The model under review builds one solid part; all positions refer to its coordinate system, in mm. Face numbers are marked on the shaded views. A direction names the side the tool comes from. Round coordinates to 2 decimals unless told otherwise and drop trailing zeros. Write each loop counter-clockwise with the first axis right and the second up, starting at its lowest first coordinate (ties: lowest second). Pieces come first, ordered by that corner, then holes. Notation, with made-up numbers: (29.5, -28) -> (68.5, -28) arc R15 ccw to (68.5, 0) -> close; hole circle Ø6 at (-6, 73.5). An arc over 180 degrees is marked (long way). Return JSON: item names as keys, results as strings. Group by question number.
1. Mouldability with a two-part tool opening along Z and no side actions: class the marked faces 1, 2 and 3 as pulls with the +Z half, pulls with the -Z half, needs draft (parallel to the pull), parting line crosses it, or undercut.
2. Take a section at C-C, the plane y = 2.45. Write out the cut boundary in (x, z).
3. Tool access review of the marked faces 4 and 5: name each direction out of +Z, -Z, +X, -X, +Y, -Y from which nothing blocks a thin tool from reaching the whole face with its end or side.
4. Take a section at D-D, the plane x = -7.25. Write out the cut boundary in (y, z), then the cut area to 3 significant figures.
5. For line 1 along X through (y, z) = (1.25, 0); line 2 along X through (y, z) = (0.7, 0.5); line 3 along Z through (x, y) = (-2.25, 2.5), list the stretches that pass through material, from the lowest coordinate up. Write a range as from..to.
6. Take a section at B-B, the plane x = 0. Write out the cut boundary in (y, z), then the cut area to 3 significant figures.
7. Take a section at A-A, the plane z = 0. Write out the cut boundary in (x, y).
8. Clearance check with flat-ended pins moving along their axes: P1, Ø2, axis at x = -7.5, y = 3.5, coming from the -Z side; P2, Ø4, axis at x = 2, z = -1.5, coming from the +Y side; P3, Ø6.5, axis at x = 0, z = 0, coming from the +Y side. State where each tip first meets the part, or that it passes through.
from build123d import *

# Parameters (mm, degrees)
SKETCH_1_R          = 10
EXTRUDE_1_DEPTH     = 5
CUT_EXTRUDE_1_DEPTH = 3
SKETCH_3_R          = 1
CUT_EXTRUDE_2_DEPTH = 3
SKETCH_5_R          = 2.5
CUT_EXTRUDE_3_DEPTH = 3


with BuildPart() as part:
    # 스케치1 → 보스-돌출1 (new body)
    with BuildSketch(Plane(origin=(0, 0, 0), x_dir=(1, 0, 0), z_dir=(0, 1, 0))):
        with Locations(Location((0, 0, 0), (0, 0, 270))):
            Circle(SKETCH_1_R)
    extrude(amount=EXTRUDE_1_DEPTH)

    # 스케치2 → 컷-돌출1 (cut)
    with BuildSketch(Plane(origin=(0, 5, 0), x_dir=(1, 0, 0), z_dir=(0, 1, 0))):
        Polygon((0, 4.618802154), (-4, 2.309401077), (-4, -2.309401077), (0, -4.618802154), (4, -2.309401077), (4, 2.309401077), align=None)
    extrude(amount=-CUT_EXTRUDE_1_DEPTH, mode=Mode.SUBTRACT)

    # 스케치3 → 컷-돌출2 (cut)
    with BuildSketch(Plane(origin=(0, 5, 0), x_dir=(1, 0, 0), z_dir=(0, 1, 0))):
        with Locations((0, 3.618802154)):
            Circle(SKETCH_3_R)
        with Locations((3.133974596, 1.809401077)):
            Circle(SKETCH_3_R)
        with Locations((3.133974596, -1.809401077)):
            Circle(SKETCH_3_R)
        with Locations((0, -3.618802154)):
            Circle(SKETCH_3_R)
        with Locations((-3.133974596, -1.809401077)):
            Circle(SKETCH_3_R)
        with Locations((-3.133974596, 1.809401077)):
            Circle(SKETCH_3_R)
    extrude(amount=-CUT_EXTRUDE_2_DEPTH, mode=Mode.SUBTRACT)

    # 스케치5 → 컷-돌출3 (cut)
    with BuildSketch(Plane.XZ):
        with Locations(Location((0, 0, 0), (0, 0, 270))):
            Circle(SKETCH_5_R)
    extrude(amount=-CUT_EXTRUDE_3_DEPTH, mode=Mode.SUBTRACT)


solid = part.part
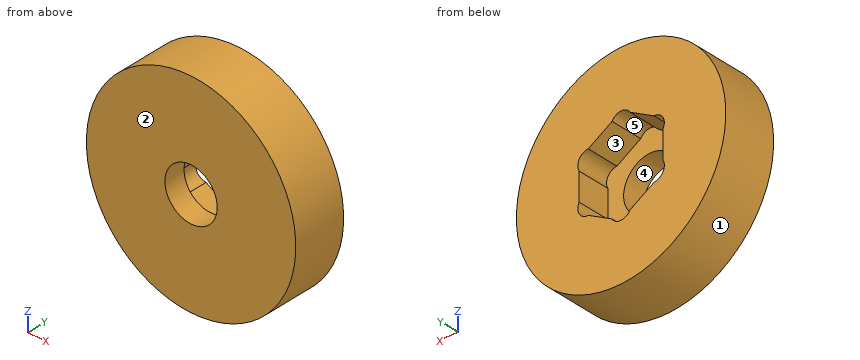
Output:
{
 "1": {"face 1": "parting line crosses it", "face 2": "needs draft", "face 3": "undercut"},
 "2": {"outline": "circle Ø20 at (0, 0); hole (-4, -1.31) arc R1 ccw to (-3.13, -2.81) -> (-0.87, -4.12) arc R1 ccw to (0.87, -4.12) -> (3.13, -2.81) arc R1 ccw to (4, -1.31) -> (4, 1.31) arc R1 ccw to (3.13, 2.81) -> (0.87, 4.12) arc R1 ccw to (-0.87, 4.12) -> (-3.13, 2.81) arc R1 ccw to (-4, 1.31) -> close"},
 "3": {"face 4": "+Y, -Y", "face 5": "+Y"},
 "4": {"outline": "(0, -6.89) -> (5, -6.89) -> (5, 6.89) -> (0, 6.89) -> close", "area": "68.9 mm^2"},
 "5": {"line 1": "x = -10..-2.5, 2.5..10", "line 2": "x = -9.99..-2.45, 2.45..9.99", "line 3": "z = -9.74..-3.32, 3.32..9.74"},
 "6": {"outline": "(0, -10) -> (5, -10) -> (5, -4.62) -> (2, -4.62) -> (2, -2.5) -> (0, -2.5) -> close; (0, 2.5) -> (2, 2.5) -> (2, 4.62) -> (5, 4.62) -> (5, 10) -> (0, 10) -> close", "area": "62.3 mm^2"},
 "7": {"outline": "(-10, 0) -> (-2.5, 0) -> (-2.5, 2) -> (-4, 2) -> (-4, 5) -> (-10, 5) -> close; (2.5, 0) -> (10, 0) -> (10, 5) -> (4, 5) -> (4, 2) -> (2.5, 2) -> close"},
 "8": {"P1": "stops at z = -7.6", "P2": "stops at y = 5", "P3": "stops at y = 2"}
}
